Here's how the part is built. I have some questions about the finished solid (model axes, mm). Face numbers are marked on the shaded views. Coordinates: 2 decimals unless noted, no trailing zeros. Write each loop counter-clockwise with the first axis right and the second up, starting at its lowest first coordinate (ties: lowest second). Pieces come first, ordered by that corner, then holes.
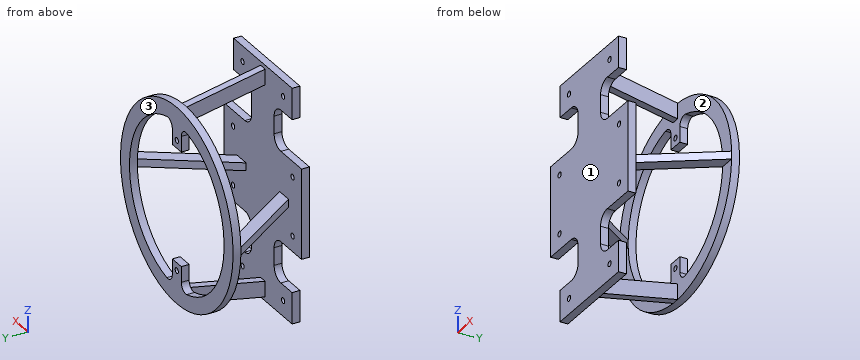
```python
from build123d import *

# Parameters (mm, degrees)
AUFSATZ_LINEAR_AUSTRAGEN1_DEPTH    = 10
SKIZZE6_R                          = 125
AUFSATZ_LINEAR_AUSTRAGEN2_DEPTH    = 10
AUFSATZ_LINEAR_AUSTRAGEN3_DEPTH    = 5
SKIZZE8_W                          = 50
SKIZZE8_H                          = 20
SCHNITT_LINEAR_AUSTRAGEN1_DEPTH    = 10
AUFSATZ_LINEAR_AUSTRAGEN4_DEPTH    = 10
SKIZZE14_W                         = 24
SKIZZE14_H                         = 115
SCHNITT_LINEAR_AUSTRAGEN2_DEPTH    = 10
SKIZZE15_W                         = 24
SKIZZE15_H                         = 115
SCHNITT_LINEAR_AUSTRAGEN3_DEPTH    = 10
AUFSATZ_LINEAR_AUSTRAGEN8_DEPTH    = 5
KERNLOCH_F_R_M8X1_0_GEWINDE2_D     = 7
KERNLOCH_F_R_M8X1_0_GEWINDE2_DEPTH = 20
KERNLOCH_F_R_M8X1_0_GEWINDE2_TIP   = 2.103012167
KERNLOCH_F_R_M8X1_0_GEWINDE3_D     = 7
KERNLOCH_F_R_M8X1_0_GEWINDE3_DEPTH = 20
KERNLOCH_F_R_M8X1_0_GEWINDE3_TIP   = 2.103012167


with BuildPart() as part:
    # Skizze1 → Aufsatz-Linear austragen1 (new body)
    with BuildSketch(Plane(origin=(0, 0, 0), x_dir=(1, 0, 0), z_dir=(0, 1, 0))):
        with BuildLine():
            Line((75.838298065, 35.851170731), (145.838298065, 35.851170731))
            Line((145.838298065, 35.851170731), (145.838298065, -79.148829269))
            Line((145.838298065, -79.148829269), (75.838298065, -79.148829269))
            ThreePointArc((75.838298065, -79.148829269), (65.231696347, -83.542227551), (60.838298065, -94.148829269))
            Line((60.838298065, -94.148829269), (60.838298065, -191.648829269))
            Line((60.838298065, -191.648829269), (10.838298065, -191.648829269))
            Line((10.838298065, -191.648829269), (10.838298065, -94.148829269))
            ThreePointArc((10.838298065, -94.148829269), (6.444899783, -83.542227551), (-4.161701935, -79.148829269))
            Line((-4.161701935, -79.148829269), (-74.161701935, -79.148829269))
            Line((-74.161701935, -79.148829269), (-74.161701935, 35.851170731))
            Line((-74.161701935, 35.851170731), (-4.161701935, 35.851170731))
            ThreePointArc((-4.161701935, 35.851170731), (6.444899783, 40.244569014), (10.838298065, 50.851170731))
            Line((10.838298065, 50.851170731), (10.838298065, 148.351170731))
            Line((10.838298065, 148.351170731), (60.838298065, 148.351170731))
            Line((60.838298065, 148.351170731), (60.838298065, 50.851170731))
            ThreePointArc((60.838298065, 50.851170731), (65.231696347, 40.244569014), (75.838298065, 35.851170731))
        make_face()
    extrude(amount=AUFSATZ_LINEAR_AUSTRAGEN1_DEPTH)



with BuildPart() as body_2:
    # Skizze6 → Aufsatz-Linear austragen2 (new body)
    with BuildSketch(Plane(origin=(0, 120, 0), x_dir=(1, 0, 0), z_dir=(0, 1, 0))):
        with Locations(Location((35.838298065, -21.648829269, 0), (0, 0, 270))):  # turned: the seam where the file's is
            Circle(SKIZZE6_R)
        with BuildLine():
            Line((25.838298065, 71.222048837), (25.838298065, 51.222048837))
            Line((25.838298065, 51.222048837), (45.838298065, 51.222048837))
            Line((45.838298065, 51.222048837), (45.838298065, 71.222048837))
            ThreePointArc((45.838298065, 71.222048837), (49.55548944, 79.001914889), (57.943561223, 80.997930742))
            ThreePointArc((57.943561223, 80.997930742), (140.838298065, -21.648829269), (57.943561223, -124.295589279))
            ThreePointArc((57.943561223, -124.295589279), (49.55548944, -122.299573426), (45.838298065, -114.519707374))
            Line((45.838298065, -114.519707374), (45.838298065, -94.519707374))
            Line((45.838298065, -94.519707374), (25.838298065, -94.519707374))
            Line((25.838298065, -94.519707374), (25.838298065, -114.519707374))
            ThreePointArc((25.838298065, -114.519707374), (22.121106689, -122.299573426), (13.733034907, -124.295589279))
            ThreePointArc((13.733034907, -124.295589279), (-69.161701935, -21.648829269), (13.733034907, 80.997930742))
            ThreePointArc((13.733034907, 80.997930742), (22.121106689, 79.001914889), (25.838298065, 71.222048837))
        make_face(mode=Mode.SUBTRACT)
    extrude(amount=-AUFSATZ_LINEAR_AUSTRAGEN2_DEPTH)


with BuildPart() as part_1:
    add(part.part)

    add(body_2.part)  # Aufsatz-Linear austragen3 merges body 2
    # Skizze7 → Aufsatz-Linear austragen3 (add, symmetric)
    with BuildSketch(Plane(origin=(35.838298065, 0, 0), x_dir=(0, 0, -1), z_dir=(1, 0, 0))):
        Polygon((-146.648829269, 110), (-126.648829269, 110), (-146.648829269, 10), (-166.648829269, 10), align=None)
    aufsatz_linear_austragen3 = extrude(amount=AUFSATZ_LINEAR_AUSTRAGEN3_DEPTH, both=True)

    # Spiegeln1: Aufsatz-Linear austragen3 across plane
    add(aufsatz_linear_austragen3.mirror(Plane.XY.offset(21.648829269)))

    # Skizze8 → Schnitt-Linear austragen1 (cut)
    with BuildSketch(Plane(origin=(0, 10, 0), x_dir=(1, 0, 0), z_dir=(0, 1, 0))):
        with Locations((35.838298065, 138.351170731)):
            Rectangle(SKIZZE8_W, SKIZZE8_H)
        with Locations((35.838298065, -181.648829269)):
            Rectangle(SKIZZE8_W, SKIZZE8_H)
    extrude(amount=-SCHNITT_LINEAR_AUSTRAGEN1_DEPTH, mode=Mode.SUBTRACT)

    # Skizze9 → Aufsatz-Linear austragen4 (add)
    with BuildSketch(Plane(origin=(0, 10, 0), x_dir=(1, 0, 0), z_dir=(0, 1, 0))):
        with BuildLine():
            Line((60.838298065, -131.648829269), (60.838298065, -171.648829269))
            Line((60.838298065, -171.648829269), (100.838298065, -171.648829269))
            Line((100.838298065, -171.648829269), (100.838298065, -131.648829269))
            Line((100.838298065, -131.648829269), (75.838298065, -131.648829269))
            ThreePointArc((75.838298065, -131.648829269), (65.231696347, -127.255430986), (60.838298065, -116.648829269))
            Line((60.838298065, -116.648829269), (60.838298065, -131.648829269))
        make_face()
        with BuildLine():
            Line((-29.161701935, -171.648829269), (10.838298065, -171.648829269))
            Line((10.838298065, -171.648829269), (10.838298065, -131.648829269))
            Line((10.838298065, -131.648829269), (10.838298065, -116.648829269))
            ThreePointArc((10.838298065, -116.648829269), (6.444899783, -127.255430986), (-4.161701935, -131.648829269))
            Line((-4.161701935, -131.648829269), (-29.161701935, -131.648829269))
            Line((-29.161701935, -131.648829269), (-29.161701935, -171.648829269))
        make_face()
        with BuildLine():
            Line((100.838298065, 128.351170731), (60.838298065, 128.351170731))
            Line((60.838298065, 128.351170731), (60.838298065, 88.351170731))
            Line((60.838298065, 88.351170731), (60.838298065, 73.351170731))
            ThreePointArc((60.838298065, 73.351170731), (65.231696347, 83.957772449), (75.838298065, 88.351170731))
            Line((75.838298065, 88.351170731), (100.838298065, 88.351170731))
            Line((100.838298065, 88.351170731), (100.838298065, 128.351170731))
        make_face()
        with BuildLine():
            Line((10.838298065, 88.351170731), (10.838298065, 128.351170731))
            Line((10.838298065, 128.351170731), (-29.161701935, 128.351170731))
            Line((-29.161701935, 128.351170731), (-29.161701935, 88.351170731))
            Line((-29.161701935, 88.351170731), (-4.161701935, 88.351170731))
            ThreePointArc((-4.161701935, 88.351170731), (6.444899783, 83.957772449), (10.838298065, 73.351170731))
            Line((10.838298065, 73.351170731), (10.838298065, 88.351170731))
        make_face()
    extrude(amount=-AUFSATZ_LINEAR_AUSTRAGEN4_DEPTH)

    # Skizze14 → Schnitt-Linear austragen2 (cut)
    with BuildSketch(Plane(origin=(0, 10, 0), x_dir=(1, 0, 0), z_dir=(0, 1, 0))):
        with Locations((133.838298065, -21.648829269)):
            Rectangle(SKIZZE14_W, SKIZZE14_H)
    extrude(amount=-SCHNITT_LINEAR_AUSTRAGEN2_DEPTH, mode=Mode.SUBTRACT)

    # Skizze15 → Schnitt-Linear austragen3 (cut)
    with BuildSketch(Plane(origin=(0, 10, 0), x_dir=(1, 0, 0), z_dir=(0, 1, 0))):
        with Locations((-62.161701935, -21.648829269)):
            Rectangle(SKIZZE15_W, SKIZZE15_H)
    extrude(amount=-SCHNITT_LINEAR_AUSTRAGEN3_DEPTH, mode=Mode.SUBTRACT)

    # Skizze16 → Aufsatz-Linear austragen8 (add, symmetric)
    with BuildSketch(Plane.XY.offset(21.648829269)):
        Polygon((-89.161701935, 110), (-69.161701935, 110), (0, 8.135310029), (-20, 8.135310029), align=None)
    aufsatz_linear_austragen8 = extrude(amount=AUFSATZ_LINEAR_AUSTRAGEN8_DEPTH, both=True)

    # Spiegeln5: Aufsatz-Linear austragen8 across plane
    add(aufsatz_linear_austragen8.mirror(Plane(origin=(35.838298065, 0, 0), x_dir=(0, 0, 1), z_dir=(1, 0, 0))))

    # Kernloch für M8x1.0 Gewinde2
    with Locations(Plane(origin=(35.838298065, 110, -61.222048837), x_dir=(0, 0, -1), z_dir=(0, -1, 0))):
        with Locations((0, 0), (-165.741756211, 0)):
            Hole(KERNLOCH_F_R_M8X1_0_GEWINDE2_D / 2, depth=KERNLOCH_F_R_M8X1_0_GEWINDE2_DEPTH)
            with Locations((0, 0, -(KERNLOCH_F_R_M8X1_0_GEWINDE2_DEPTH + KERNLOCH_F_R_M8X1_0_GEWINDE2_TIP / 2))):  # 118° drill point
                Cone(0, KERNLOCH_F_R_M8X1_0_GEWINDE2_D / 2, KERNLOCH_F_R_M8X1_0_GEWINDE2_TIP, mode=Mode.SUBTRACT)

    # Kernloch für M8x1.0 Gewinde3
    with Locations(Plane(origin=(101.838298065, 10, -15.851170731), x_dir=(0, 0, 1), z_dir=(0, 1, 0))):
        with Locations((0, 0), (75, 0), (0, -132), (-92.5, -111), (75, -132), (167.5, -111), (167.5, -21), (-92.5, -21)):
            Hole(KERNLOCH_F_R_M8X1_0_GEWINDE3_D / 2, depth=KERNLOCH_F_R_M8X1_0_GEWINDE3_DEPTH)
            with Locations((0, 0, -(KERNLOCH_F_R_M8X1_0_GEWINDE3_DEPTH + KERNLOCH_F_R_M8X1_0_GEWINDE3_TIP / 2))):  # 118° drill point
                Cone(0, KERNLOCH_F_R_M8X1_0_GEWINDE3_D / 2, KERNLOCH_F_R_M8X1_0_GEWINDE3_TIP, mode=Mode.SUBTRACT)


solid = part_1.part
```
1) Imagine slicing it at B-B on y = 42. Please give me the cut outline in (x, z), then the cut area to 3 significant figures.
Values follow:
outline: (-42.99, 16.65) - (-22.99, 16.65) - (-22.99, 26.65) - (-42.99, 26.65) - close; (30.84, -116.95) - (40.84, -116.95) - (40.84, -96.95) - (30.84, -96.95) - close; (30.84, 140.25) - (40.84, 140.25) - (40.84, 160.25) - (30.84, 160.25) - close; (94.67, 16.65) - (114.67, 16.65) - (114.67, 26.65) - (94.67, 26.65) - close
area: 800 mm2
2) I need wall thicknesses on probe 1 along Y at (x, z) = (60.5, 124); probe 2 along Y at (x, z) = (-78.5, -7.5); probe 3 along Y at (x, z) = (106.5, -14.5). Which ranges of each line are inside material? Lowest first, please.
Values follow:
probe 1: y = 0 to 10, 110 to 120
probe 2: y = 110 to 120
probe 3: y = 0 to 10
3) We'd pull the mould along Y, two halves only. Please class the marked faces 1, 2 and 3: pulls with the +Y half, pulls with the -Y half, needs draft (parallel to the pull), parting line crosses it, or undercut.
Values follow:
face 1: pulls with the -Y half
face 2: undercut
face 3: pulls with the +Y half
4) Imagine slicing it at D-D on x = 6.5. Please give me the cut outline in (y, z).
Values follow:
outline: (0, -128.35) - (10, -128.35) - (10, -83.9) - (0, -83.9) - close; (0, -40.3) - (10, -40.3) - (10, 83.6) - (0, 83.6) - close; (0, 127.2) - (10, 127.2) - (10, 171.65) - (0, 171.65) - close; (110, -99.86) - (120, -99.86) - (120, -79.17) - (110, -79.17) - close; (110, 122.47) - (120, 122.47) - (120, 143.16) - (110, 143.16) - close
5) Imagine slicing it at C-C on z = -32.5. Please give me the cut outline in (x, y), then the cut area to 3 significant figures.
Values follow:
outline: (-76.82, 110) - (-54.12, 110) - (-54.12, 120) - (-76.82, 120) - close; (-50.16, 0) - (121.84, 0) - (121.84, 10) - (-50.16, 10) - close; (125.8, 110) - (148.5, 110) - (148.5, 120) - (125.8, 120) - close
area: 2,170 mm2
6) Will these pins go through, and if not, where does the flat tip stop? pin 1 (8 mm diameter, centred on y = 4, z = -100.5, fed in from +X); pin 2 (6 mm diameter, centred on x = -3, z = -24.5, fed in from +Y); pin 3 (3 mm diameter, centred on y = 6.5, z = -4, fed in from +X); pin 4 (10 mm diameter, centred on y = 86.5, z = 124.5, fed in from -X).
Values follow:
pin 1: stops at x = 100.84
pin 2: stops at y = 10
pin 3: stops at x = 121.84
pin 4: passes through
7) Imagine slicing it at A-A on x = -57. Please give me the cut outline in (y, z), then the cut area to 3 significant figures.
Values follow:
outline: (62.63, 16.65) - (92.09, 16.65) - (92.09, 26.65) - (62.63, 26.65) - close; (110, -62.05) - (120, -62.05) - (120, -27.4) - (110, -27.4) - close; (110, 70.7) - (120, 70.7) - (120, 105.35) - (110, 105.35) - close
area: 988 mm2
